Geometry check sheet. Reference: the model listing, model coordinates, mm. Coordinates: 2 decimals unless noted, no trailing zeros. Answer in a Markdown table with one row per item. Add a question column.
Q1. Section check A-A, the plane y = 0.6. Count the separate pieces of the cut face and the enclosed holes in it, and give its area (3 significant figures).
Q2. Thickness scan on line 1 (X direction, y = 2.85, z = 10.5) (3 decimals); line 2 (X direction, y = 1.7, z = -123.19); line 3 (X direction, y = 2.25, z = -139.7). Record the ranges inside material, lowest first.
Q3. Gauge pin test, flat end, axial feed: P1, Ø11.5, axis at x = -19.05, z = -139.7, coming from the -Y side. Record the tip position at first contact, or that the pin passes through.
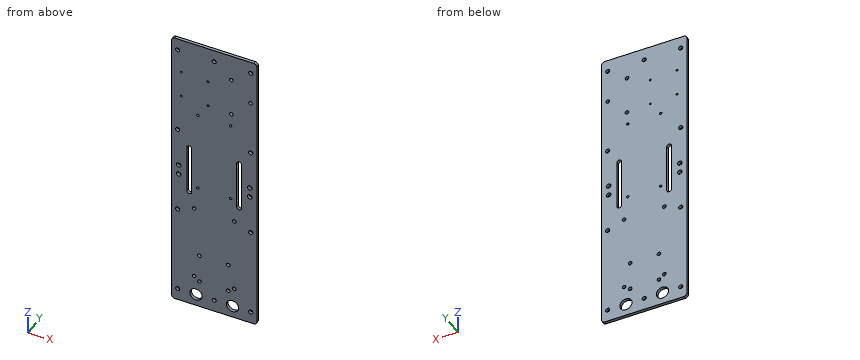
```python
from build123d import *

# Parameters (mm, degrees)
PLATE_THICKNESS_DEPTH        = 3.175
SKETCH3_R                    = 2.159
MOUNTING_HOLES_DEPTH         = 159.781746826
SKETCH4_R                    = 1.905
JETSON_HOLES_W_O_MOUNT_DEPTH = 159.781746826
SKETCH5_R                    = 1.905
PDB_HOLES_DEPTH              = 159.781746826
SKETCH7_R                    = 1.27
PIXHAWK_HOLES_DEPTH          = 159.781746826
BATTERY_HOLES_DEPTH          = 159.781746826
VENTRAL_CAMERA_HOLES_REACH   = 160.782
SKETCH10_R                   = 1
SKETCH12_R                   = 6.35
WIFI_ANTENNA_HOLES_DEPTH     = 159.781746826
SKETCH6_R                    = 1.905
TERARANGER_HOLES_DEPTH       = 159.781746826
SKETCH14_R                   = 2.38125
SONARHOLES_DEPTH             = 159.781746826


with BuildPart() as part:
    # Sketch2 → Plate Thickness (new body)
    with BuildSketch(Plane(origin=(0, 0, 0), x_dir=(1, 0, 0), z_dir=(0, 1, 0))):
        with BuildLine():
            Line((-41.275, 152.4), (41.275, 152.4))
            ThreePointArc((41.275, 152.4), (43.52006403, 151.47006403), (44.45, 149.225))
            Line((44.45, 149.225), (44.45, -149.225))
            ThreePointArc((44.45, -149.225), (43.52006403, -151.47006403), (41.275, -152.4))
            Line((41.275, -152.4), (-41.275, -152.4))
            ThreePointArc((-41.275, -152.4), (-43.52006403, -151.47006403), (-44.45, -149.225))
            Line((-44.45, -149.225), (-44.45, 149.225))
            ThreePointArc((-44.45, 149.225), (-43.52006403, 151.47006403), (-41.275, 152.4))
        make_face()
    extrude(amount=PLATE_THICKNESS_DEPTH)

    # Sketch3 → Mounting holes (cut, through all)
    with BuildSketch(Plane(origin=(0, 3.175, 0), x_dir=(1, 0, 0), z_dir=(0, 1, 0))):
        with Locations(Location((-38.1, 139.7, 0), (0, 0, 270))):
            Circle(SKETCH3_R)
        with Locations(Location((-38.1, 46.566666666, 0), (0, 0, 270))):
            Circle(SKETCH3_R)
        with Locations(Location((-38.1, -46.56666582, 0), (0, 0, 90))):
            Circle(SKETCH3_R)
        with Locations(Location((-38.1, -139.7, 0), (0, 0, 90))):
            Circle(SKETCH3_R)
        with Locations(Location((38.1, -139.7, 0), (0, 0, 270))):
            Circle(SKETCH3_R)
        with Locations(Location((38.1, -46.56666582, 0), (0, 0, 270))):
            Circle(SKETCH3_R)
        with Locations(Location((38.1, 46.566666666, 0), (0, 0, 90))):
            Circle(SKETCH3_R)
        with Locations(Location((38.1, 139.7, 0), (0, 0, 90))):
            Circle(SKETCH3_R)
        with Locations(Location((0, 139.7, 0), (0, 0, 270))):
            Circle(SKETCH3_R)
        with Locations(Location((0, -139.7, 0), (0, 0, 90))):
            Circle(SKETCH3_R)
    extrude(amount=-MOUNTING_HOLES_DEPTH, mode=Mode.SUBTRACT)

    # Sketch4 → Jetson Holes (w/o mount) (cut, through all)
    with BuildSketch(Plane(origin=(0, 3.175, 0), x_dir=(1, 0, 0), z_dir=(0, 1, 0))):
        with Locations(Location((-21.0058, 118.808268359, 0), (0, 0, 270))):
            Circle(SKETCH4_R)
        with Locations(Location((-21.0058, 39.814268359, 0), (0, 0, 270))):
            Circle(SKETCH4_R)
        with Locations(Location((21.0058, 39.814268359, 0), (0, 0, 90))):
            Circle(SKETCH4_R)
        with Locations(Location((21.0058, 118.808268359, 0), (0, 0, 90))):
            Circle(SKETCH4_R)
    extrude(amount=-JETSON_HOLES_W_O_MOUNT_DEPTH, mode=Mode.SUBTRACT)

    # Sketch5 → PDB holes (cut, through all)
    with BuildSketch(Plane(origin=(0, 3.175, 0), x_dir=(1, 0, 0), z_dir=(0, 1, 0))):
        with Locations(Location((-15.378405846, 123.19, 0), (0, 0, 270))):
            Circle(SKETCH5_R)
        with Locations(Location((14.618994154, 123.19, 0), (0, 0, 270))):
            Circle(SKETCH5_R)
        with Locations(Location((14.618994154, 93.1926, 0), (0, 0, 270))):
            Circle(SKETCH5_R)
        with Locations(Location((-15.378405846, 93.1926, 0), (0, 0, 270))):
            Circle(SKETCH5_R)
    extrude(amount=-PDB_HOLES_DEPTH, mode=Mode.SUBTRACT)

    # Sketch7 → PixHawk Holes (cut, through all)
    with BuildSketch(Plane(origin=(0, 3.175, 0), x_dir=(1, 0, 0), z_dir=(0, 1, 0))):
        with Locations(Location((-17.145, 14.489268954, 0), (0, 0, 270))):
            Circle(SKETCH7_R)
        with Locations(Location((-17.145, -70.600731046, 0), (0, 0, 270))):
            Circle(SKETCH7_R)
        with Locations(Location((17.145, -70.600731046, 0), (0, 0, 270))):
            Circle(SKETCH7_R)
        with Locations(Location((17.145, 14.489268954, 0), (0, 0, 270))):
            Circle(SKETCH7_R)
    extrude(amount=-PIXHAWK_HOLES_DEPTH, mode=Mode.SUBTRACT)

    # Sketch8 → Battery Holes (cut, through all)
    with BuildSketch(Plane(origin=(0, 3.175, 0), x_dir=(1, 0, 0), z_dir=(0, 1, 0))):
        with BuildLine():
            Line((-23.495, 21.689654687), (-23.495, -29.110345313))
            ThreePointArc((-23.495, -29.110345313), (-26.035, -31.650345313), (-28.575, -29.110345313))
            Line((-28.575, -29.110345313), (-28.575, 21.689654687))
            ThreePointArc((-28.575, 21.689654687), (-26.035, 24.229654687), (-23.495, 21.689654687))
        make_face()
        with BuildLine():
            Line((23.495, 21.689654687), (23.495, -29.110345313))
            ThreePointArc((23.495, -29.110345313), (26.035, -31.650345313), (28.575, -29.110345313))
            Line((28.575, -29.110345313), (28.575, 21.689654687))
            ThreePointArc((28.575, 21.689654687), (26.035, 24.229654687), (23.495, 21.689654687))
        make_face()
    extrude(amount=-BATTERY_HOLES_DEPTH, mode=Mode.SUBTRACT)

    # Sketch10 → Ventral Camera holes (cut, up to next)
    with BuildSketch(Plane(origin=(0, 3.175, 0), x_dir=(1, 0, 0), z_dir=(0, 1, 0)), mode=Mode.PRIVATE) as ventral_camera_holes_sk1:
        with Locations(Location((-34.315460092, -87.008641581, 0), (0, 0, 270))):
            Circle(SKETCH10_R)
    ventral_camera_holes_tool1 = extrude(ventral_camera_holes_sk1.sketch, amount=-VENTRAL_CAMERA_HOLES_REACH, mode=Mode.PRIVATE) & part.part
    # Sketch10 → Ventral Camera holes (cut, up to next)
    with BuildSketch(Plane(origin=(0, 3.175, 0), x_dir=(1, 0, 0), z_dir=(0, 1, 0)), mode=Mode.PRIVATE) as ventral_camera_holes_sk2:
        with Locations(Location((-34.29, -115.008630005, 0), (0, 0, 270))):
            Circle(SKETCH10_R)
    ventral_camera_holes_tool2 = extrude(ventral_camera_holes_sk2.sketch, amount=-VENTRAL_CAMERA_HOLES_REACH, mode=Mode.PRIVATE) & part.part
    # Sketch10 → Ventral Camera holes (cut, up to next)
    with BuildSketch(Plane(origin=(0, 3.175, 0), x_dir=(1, 0, 0), z_dir=(0, 1, 0)), mode=Mode.PRIVATE) as ventral_camera_holes_sk3:
        with Locations(Location((-6.316568972, -85.789139736, 0), (0, 0, 270))):
            Circle(SKETCH10_R)
    ventral_camera_holes_tool3 = extrude(ventral_camera_holes_sk3.sketch, amount=-VENTRAL_CAMERA_HOLES_REACH, mode=Mode.PRIVATE) & part.part
    # Sketch10 → Ventral Camera holes (cut, up to next)
    with BuildSketch(Plane(origin=(0, 3.175, 0), x_dir=(1, 0, 0), z_dir=(0, 1, 0)), mode=Mode.PRIVATE) as ventral_camera_holes_sk4:
        with Locations(Location((-6.316568972, -113.789139736, 0), (0, 0, 270))):
            Circle(SKETCH10_R)
    ventral_camera_holes_tool4 = extrude(ventral_camera_holes_sk4.sketch, amount=-VENTRAL_CAMERA_HOLES_REACH, mode=Mode.PRIVATE) & part.part
    add(ventral_camera_holes_tool1.solids().sort_by_distance((-34.31546, 3.175, 87.008642))[0], mode=Mode.SUBTRACT)
    add(ventral_camera_holes_tool2.solids().sort_by_distance((-34.29, 3.175, 115.00863))[0], mode=Mode.SUBTRACT)
    add(ventral_camera_holes_tool3.solids().sort_by_distance((-6.316569, 3.175, 85.78914))[0], mode=Mode.SUBTRACT)
    add(ventral_camera_holes_tool4.solids().sort_by_distance((-6.316569, 3.175, 113.78914))[0], mode=Mode.SUBTRACT)

    # Sketch12 → Wifi antenna holes (cut, through all)
    with BuildSketch(Plane(origin=(0, 3.175, 0), x_dir=(1, 0, 0), z_dir=(0, 1, 0))):
        with Locations(Location((-19.05, 139.7, 0), (0, 0, 270))):
            Circle(SKETCH12_R)
        with Locations(Location((19.05, 139.7, 0), (0, 0, 270))):
            Circle(SKETCH12_R)
    extrude(amount=-WIFI_ANTENNA_HOLES_DEPTH, mode=Mode.SUBTRACT)

    # Sketch6 → TeraRanger Holes (cut, through all)
    with BuildSketch(Plane(origin=(0, 3.175, 0), x_dir=(1, 0, 0), z_dir=(0, 1, 0))):
        with Locations(Location((37.917522463, -104.394, 0), (0, 0, 270))):
            Circle(SKETCH6_R)
        with Locations(Location((17.917522463, -84.46, 0), (0, 0, 270))):
            Circle(SKETCH6_R)
        with Locations(Location((17.917522463, -124.46, 0), (0, 0, 270))):
            Circle(SKETCH6_R)
    extrude(amount=-TERARANGER_HOLES_DEPTH, mode=Mode.SUBTRACT)

    # Sketch14 → Sonarholes (cut, through all)
    with BuildSketch(Plane(origin=(0, 3.175, 0), x_dir=(1, 0, 0), z_dir=(0, 1, 0))):
        with Locations(Location((-37.138013211, 5.246249985, 0), (0, 0, 270))):
            Circle(SKETCH14_R)
        with Locations(Location((-37.138013211, -5.246249985, 0), (0, 0, 90))):
            Circle(SKETCH14_R)
        with Locations(Location((37.138013211, -5.246249985, 0), (0, 0, 270))):
            Circle(SKETCH14_R)
        with Locations(Location((37.138013211, 5.246249985, 0), (0, 0, 90))):
            Circle(SKETCH14_R)
    extrude(amount=-SONARHOLES_DEPTH, mode=Mode.SUBTRACT)


solid = part.part
```
Calculated:
| question | item | result |
|---|---|---|
| 1 | separate pieces | 1 |
| 1 | enclosed holes | 37 |
| 1 | area | 25,900 mm² |
| 2 | line 1 | x = -44.45 to -28.575, -23.495 to 23.495, 28.575 to 44.45 |
| 2 | line 2 | x = -44.45 to -17.28, -13.47 to 12.71, 16.52 to 44.45 |
| 2 | line 3 | x = -44.45 to -40.26, -35.94 to -25.4, -12.7 to -2.16, 2.16 to 12.7, 25.4 to 35.94, 40.26 to 44.45 |
| 3 | P1 | passes through |
